```python
from build123d import *

# Parameters (mm, degrees)
SKETCH1_R             = 12.5
BOSS_EXTRUDE2_DEPTH   = 35
SKETCH6_R             = 17.5
BOSS_EXTRUDE3_DEPTH   = 10
BOSS_EXTRUDE4_START   = 50
SKETCH7_R             = 12.5
BOSS_EXTRUDE4_DEPTH   = 50
SKETCH8_R             = 10
BOSS_EXTRUDE5_DEPTH   = 40
CHAMFER1_SIZE         = 1
CUT_EXTRUDE11_START   = 5.24705599
CUT_EXTRUDE11_DEPTH   = 8.75294401
CUT_EXTRUDE11_START_2 = 6
CUT_EXTRUDE11_2_DEPTH = 28


with BuildPart() as part:
    # Sketch1 → Boss-Extrude2 (new body)
    with BuildSketch(Plane.XY):
        Circle(SKETCH1_R)
    extrude(amount=BOSS_EXTRUDE2_DEPTH)

    # Sketch6 → Boss-Extrude3 (add)
    with BuildSketch(Plane(origin=(0, 0, 0), x_dir=(-1, 0, 0), z_dir=(0, 0, -1))):
        Circle(SKETCH6_R)
    extrude(amount=BOSS_EXTRUDE3_DEPTH)

    # Sketch7 → Boss-Extrude4 (add)
    with BuildSketch(Plane(origin=(0, 0, -10), x_dir=(-1, 0, 0), z_dir=(0, 0, -1)).offset(BOSS_EXTRUDE4_START)):
        with Locations(Location((0, 0, 0), (0, 0, 180))):
            Circle(SKETCH7_R)
    extrude(amount=-BOSS_EXTRUDE4_DEPTH)

    # Sketch8 → Boss-Extrude5 (add)
    with BuildSketch(Plane(origin=(0, 0, -60), x_dir=(-1, 0, 0), z_dir=(0, 0, -1))):
        Circle(SKETCH8_R)
    extrude(amount=BOSS_EXTRUDE5_DEPTH)

    # Chamfer1
    chamfer1_edges = [part.edges().sort_by_distance(p)[0] for p in [
        (-12.5, 0, -60),
        (10, 0, -100),
        (-12.5, 0, 35),
        (17.5, 0, 0),
        (17.5, 0, -10),
    ]]
    chamfer(chamfer1_edges, length=CHAMFER1_SIZE)

    # Cut-Extrude11: read off the stored shape, not the designer's step
    # Cut-Extrude11 outline → Cut-Extrude11 (cut)
    with BuildSketch(Plane(origin=(0, 0, 0), x_dir=(0, 0, -1), z_dir=(1, 0, 0)).offset(CUT_EXTRUDE11_START)):
        with BuildLine():
            Line((-10, 2.501922686), (-30, 2.501922686))
            add(Edge.make_bspline(
                [(-30, 2.501922686), (-30.662861656, 2.501922686), (-31.308912406, 2.229348378), (-32.229370531, 1.308874674), (-32.501390649, 0.6564432), (-32.502453075, -0.652381374), (-32.23483126, -1.302936015), (-31.305267278, -2.233470473), (-30.662865998, -2.501922686), (-30, -2.501922686)],
                knots=[0, 0, 0, 0, 0.25, 0.25, 0.5, 0.5, 0.75, 0.75, 1, 1, 1, 1], degree=3))
            Line((-30, -2.501922686), (-10, -2.501922686))
            add(Edge.make_bspline(
                [(-10, -2.501922686), (-9.337138344, -2.501922686), (-8.691087594, -2.229348378), (-7.770629469, -1.308874674), (-7.498609351, -0.6564432), (-7.497546925, 0.652381374), (-7.76516874, 1.302936015), (-8.694732722, 2.233470473), (-9.337134002, 2.501922686), (-10, 2.501922686)],
                knots=[0, 0, 0, 0, 0.25, 0.25, 0.5, 0.5, 0.75, 0.75, 1, 1, 1, 1], degree=3))
        make_face()
    extrude(amount=CUT_EXTRUDE11_DEPTH, mode=Mode.SUBTRACT)

    # Cut-Extrude11 2 outline → Cut-Extrude11 2 (add)
    with BuildSketch(Plane.XY.offset(CUT_EXTRUDE11_START_2)):
        with BuildLine():
            ThreePointArc((5.24705609, -2.501922686), (5.5, 0), (5.24705609, 2.501922686))
            Line((5.24705609, 2.501922686), (5.24705609, -2.501922686))
        make_face()
    extrude(amount=CUT_EXTRUDE11_2_DEPTH)


solid = part.part
```
CAD build for the part. Positions are in the model's coordinates, mm. A direction names the side the tool comes from. Coordinates: 2 decimals unless noted, no trailing zeros. Order: outer loops, then holes, each group sorted by start corner. A loop starts at its lowest first (then second) coordinate and runs counter-clockwise, first axis right, second up.
(1) Pin check, flat tips, straight feed: pin 1 Ø2 at (x, z) = (9, 16) entering from +Y; pin 2 Ø7.5 at (x, z) = (9.5, 25) entering from -Y; pin 3 Ø1 at (y, z) = (2.5, -48.5) entering from -X. Stop position of each tip, or through.
Solution:
pin 1: stops at y = 9.6
pin 2: stops at y = -11.1
pin 3: stops at x = -12.34
(2) Drill centre lines: L1, parallel to Z at x = -10.5, y = -11.5; L2, parallel to Y at x = 10.5, z = 27.5; L3, parallel to Z at x = -8.5, y = 6. Where is each one in solid material? Low to high.
Solution:
L1: z = -10 to 0
L2: y = -6.78 to -2.5, 2.5 to 6.78
L3: z = -60 to 35
(3) Saw through at C-C, the plane z = -19.5. Write the cut outline in (x, y).
Solution:
outline: circle Ø25 at (0, 0)
(4) Saw through at B-B, the plane z = -82. Write the cut outline in (x, y), and give its area (3 significant figures).
Solution:
outline: circle Ø20 at (0, 0)
area: 314 mm2
(5) Saw through at A-A, the plane x = 0. Write the cut outline in (y, z), and give its area (3 significant figures).
Solution:
outline: (-17.5, -9) - (-16.5, -10) - (-12.5, -10) - (-12.5, -59) - (-11.5, -60) - (-10, -60) - (-10, -99) - (-9, -100) - (9, -100) - (10, -99) - (10, -60) - (11.5, -60) - (12.5, -59) - (12.5, -10) - (16.5, -10) - (17.5, -9) - (17.5, -1) - (16.5, 0) - (12.5, 0) - (12.5, 34) - (11.5, 35) - (-11.5, 35) - (-12.5, 34) - (-12.5, 0) - (-16.5, 0) - (-17.5, -1) - close
area: 3,270 mm2
(6) Which spindle directions (+Z, -Z, +X, -X, +Y, -Y) get a long thin tool onto all of the face, cutting with end or side? Do faces 1 (the face through (13.887, -10.648, -4.944)), 2 (the face through (9, 2.502, 20)), 3 (the face through (-9, -5, -60)), 4 (the face through (11.923, 3.755, 16.762)). Say none if no direction does.
Solution:
face 1: +Z, -Z
face 2: +X
face 3: -Z
face 4: +Z
(7) Mould opens along Z. For faces 5 (the face through (5.5, 0, 19.8)), 6 (the face through (0, 0, 35)), 7 (the face through (12.3, 3.7, -10)), 8 (the face through (2.17, -9.76, -79.23)) say: released by +Z, released by -Z, zero draft, split by the parting line, or undercut.
Solution:
face 5: undercut
face 6: released by +Z
face 7: released by -Z
face 8: zero draft
